The model under review builds one solid part; all positions refer to its coordinate system, in mm. A direction names the side the tool comes from. Round coordinates to 2 decimals unless told otherwise and drop trailing zeros. Order: outer loops, then holes, each group sorted by start corner. A loop starts at its lowest first (then second) coordinate and runs counter-clockwise, first axis right, second up.
1) Clearance check with flat-ended pins moving along their axes: P1, Ø2, axis at y = -2.5, z = 0.5, coming from the +X side; P2, Ø2, axis at y = 1, z = 0, coming from the -X side; P3, Ø7, axis at x = 9, y = -7.5, coming from the +Z side. State where each tip first meets the part, or that it passes through.
2) Consider section C-C (z = -0.75). Give the boundary of the cut face in (x, y).
3) Consider section A-A (y = 0). Give the boundary of the cut face in (x, z), then the cut area to 3 significant figures.
4) Consider section B-B (x = -10.5). Give the boundary of the cut face in (y, z).
5) Machinability: for faces 1 (the face through (7.5, -6, 0)), 2 (the face through (-6.5, 0, 0)), 3 (the face through (10.07, -14.27, -0.03)), which of the approach directions +Z, -Z, +X, -X, +Y, -Y give a long, thin tool a straight path to every point of the face, cutting with its end or side? Answer none if there is none.
6) To check wall thickness, follow L1, parallel to Y at x = -10.5, z = 2.5; L2, parallel to Z at x = -12.5, y = 0.25; L3, parallel to Z at x = 7.5, y = 0.75. State the ranges of each line that lie inside material, in increasing order.
7) Consider section D-D (x = 4.5). Give the boundary of the cut face in (y, z), then the cut area to 3 significant figures.
8) Mouldability with a two-part tool opening along X and no side actions: class faces 4 (the face through (-8.976, -0.632, -2.859)), 5 (the face through (11.22, -13.81, 0.03)), 6 (the face through (-14, 0, 3)), 7 (the face through (8, -5, 2)) as pulls with the +X half, pulls with the -X half, needs draft (parallel to the pull), parting line crosses it, or undercut.
from build123d import *

# Parameters (mm, degrees)
SKETCH1_W           = 13
SKETCH1_H           = 7
BOSS_EXTRUDE1_DEPTH = 3.5
SKETCH3_W           = 7.5
SKETCH3_H           = 7
BOSS_EXTRUDE2_DEPTH = 1.3
CUT_EXTRUDE2_REACH  = 18.039
SKETCH4_R           = 1.65
FILLET3_R           = 0.7
FILLET4_R           = 2
BOSS_EXTRUDE4_DEPTH = 2
FILLET5_R           = 1


with BuildPart() as part:
    # Sketch1 → Boss-Extrude1 (new, symmetric)
    with BuildSketch(Plane.XY):
        Rectangle(SKETCH1_W, SKETCH1_H)
    extrude(amount=BOSS_EXTRUDE1_DEPTH, both=True)

    # Sketch3 → Boss-Extrude2 (add)
    with BuildSketch(Plane.XY.offset(3.5)):
        with Locations((-10.25, 0)):
            Rectangle(SKETCH3_W, SKETCH3_H)
    boss_extrude2 = extrude(amount=-BOSS_EXTRUDE2_DEPTH)

    # Sketch4 → Cut-Extrude2 (cut, up to next)
    with BuildSketch(Plane.XY.offset(3.5), mode=Mode.PRIVATE) as cut_extrude2_sk1:
        with Locations((-10.5, 0)):
            Circle(SKETCH4_R)
    cut_extrude2_tool1 = extrude(cut_extrude2_sk1.sketch, amount=-CUT_EXTRUDE2_REACH, mode=Mode.PRIVATE) & part.part
    cut_extrude2 = cut_extrude2_tool1.solids().sort_by_distance((-10.5, 0, 3.5))[0]
    add(cut_extrude2, mode=Mode.SUBTRACT)

    # Mirror1: Boss-Extrude2, Cut-Extrude2 across plane
    add(boss_extrude2.mirror(Plane.XY))
    add(cut_extrude2.mirror(Plane.XY), mode=Mode.SUBTRACT)

    # Fillet3
    fillet3_edges = [part.edges().sort_by_distance(p)[0] for p in [
        (-6.5, -3.5, 0),
    ]]
    fillet(fillet3_edges, radius=FILLET3_R)

    # Fillet4
    fillet4_edges = [part.edges().sort_by_distance(p)[0] for p in [
        (-14, -3.5, 2.85),
        (-14, 3.5, 2.85),
        (-14, 3.5, -2.85),
        (-14, -3.5, -2.85),
    ]]
    fillet(fillet4_edges, radius=FILLET4_R)

    # Sketch6 → Boss-Extrude4 (add, symmetric)
    with BuildSketch(Plane.XY):
        Polygon((6.5, 3.5), (9, 3.5), (9, -8.039733235), (12.441458618, -12.9546455), (9.984002485, -14.675374809), (5.8, -8.7), (5.8, -7.7), (7.5, -7.7), (7.5, -3.5), (6.5, -3.5), align=None)
    extrude(amount=BOSS_EXTRUDE4_DEPTH, both=True)

    # Fillet5
    fillet5_edges = [part.edges().sort_by_distance(p)[0] for p in [
        (7.5, -3.5, 0),
        (7.5, -7.7, 0),
        (5.8, -8.7, 0),
        (9.984002485, -14.675374809, 0),
        (12.441458618, -12.9546455, 0),
        (9, -8.039733235, 0),
    ]]
    fillet(fillet5_edges, radius=FILLET5_R)


solid = part.part
Answer below:
1. P1: stops at x = 9
1. P2: stops at x = -6.5
1. P3: stops at z = 2
2. outline: (-6.5, -2.8) arc R0.7 ccw to (-5.8, -3.5) - (6.5, -3.5) arc R1 cw to (7.5, -4.5) - (7.5, -6.7) arc R1 cw to (6.5, -7.7) - (5.8, -7.7) - (5.8, -8.38) arc R1 ccw to (5.98, -8.96) - (9.41, -13.86) arc R1 ccw to (10.8, -14.1) - (11.62, -13.53) arc R1 ccw to (11.87, -12.14) - (9.18, -8.3) arc R1 cw to (9, -7.72) - (9, 3.5) - (-6.5, 3.5) - close
3. outline: (-14, -3.5) - (-12.15, -3.5) - (-12.15, -2.2) - (-14, -2.2) - close; (-14, 2.2) - (-12.15, 2.2) - (-12.15, 3.5) - (-14, 3.5) - close; (-8.85, -3.5) - (6.5, -3.5) - (6.5, -2) - (9, -2) - (9, 2) - (6.5, 2) - (6.5, 3.5) - (-8.85, 3.5) - (-8.85, 2.2) - (-6.5, 2.2) - (-6.5, -2.2) - (-8.85, -2.2) - close
3. area: 112 mm2
4. outline: (-3.5, -3.5) - (-1.65, -3.5) - (-1.65, -2.2) - (-3.5, -2.2) - close; (-3.5, 2.2) - (-1.65, 2.2) - (-1.65, 3.5) - (-3.5, 3.5) - close; (1.65, -3.5) - (3.5, -3.5) - (3.5, -2.2) - (1.65, -2.2) - close; (1.65, 2.2) - (3.5, 2.2) - (3.5, 3.5) - (1.65, 3.5) - close
5. face 1: +Z, -Z, -X
5. face 2: -X, +Y, -Y
5. face 3: +Z, -Z, -Y
6. L1: y = -3.5 to -1.65, 1.65 to 3.5
6. L2: z = -3.5 to -2.2, 2.2 to 3.5
6. L3: z = -2 to 2
7. outline: (-3.5, -3.5) - (3.5, -3.5) - (3.5, 3.5) - (-3.5, 3.5) - close
7. area: 49.0 mm2
8. face 4: undercut
8. face 5: pulls with the +X half
8. face 6: pulls with the -X half
8. face 7: needs draft
